The listing builds one solid part. Answer for the finished solid, in the listing's coordinates (mm). A direction names the side the tool comes from. Coordinates: 2 decimals unless noted, no trailing zeros. Write each loop counter-clockwise with the first axis right and the second up, starting at its lowest first coordinate (ties: lowest second). Pieces come first, ordered by that corner, then holes. Notation, with made-up numbers: M -7.75,9.25 L 33.25,9.25 A31 cw 33.25,43.25 Z; hole C 86,-35 d6. An arc over 180 degrees is marked long. Answer as a JSON object with one key per item and string values. Group by question number.
from build123d import *

# Parameters (mm, degrees)
F0_W      = 140
F0_H      = 70
F1_DEPTH  = 37
F2_W      = 138
F2_H      = 35
F3_DEPTH  = 70.001
F5_D      = 3.3
F6_W      = 2
F6_H      = 35
F7_DEPTH  = 35
F8_SIZE   = 34.99999
F10_DEPTH = 70.001
F11_W     = 60
F11_H     = 13
F12_DEPTH = 2.001
F13_W     = 33.65
F13_H     = 21.7
F13_W_2   = 26.7
F13_H_2   = 19.15
F13_W_3   = 30.8
F13_W_4   = 16.7
F13_W_5   = 22.15
F14_DEPTH = 2.001
F15_R     = 5
F17_D     = 4.4


# Not quite as in the source:
# - a fillet or chamfer is up to 0.001 mm smaller than in the source, because OpenCascade refuses the exact size
# - a feature names something its author has since deleted; it is built from what else it names


with BuildPart() as f1:
    # F0 (on Top) → F1 (new body)
    with BuildSketch(Plane.XY):
        with Locations((-10, 0)):
            Rectangle(F0_W, F0_H)
    extrude(amount=F1_DEPTH)

    # F2 (on face) → F3 (cut, through all)
    with BuildSketch(Plane.XZ.offset(35)):
        with Locations((-11, 19.5)):
            Rectangle(F2_W, F2_H)
    extrude(amount=-F3_DEPTH, mode=Mode.SUBTRACT)

    # F5 (through all)
    with Locations(Plane.XY.offset(2)):
        with Locations((-67, 25), (-59.5, 17.5), (-67, -25), (-59.5, -17.5), (-29.5, -17.5), (-22, -25), (-12, -20), (-12, 20), (-22, 25), (-29.5, 17.5), (28, 20), (38, 20), (38, -20), (28, -20)):
            Hole(F5_D / 2)

    # F6 (on face) → F7 (join)
    with BuildSketch(Plane(origin=(58, 0, 0), x_dir=(0, -1, 0), z_dir=(-1, 0, 0))):
        with Locations((-34, 19.5)):
            Rectangle(F6_W, F6_H)
        with Locations((34, 19.5)):
            Rectangle(F6_W, F6_H)
    extrude(amount=F7_DEPTH)

    # F8 (size 35 in the source; OpenCascade refuses exactly that, so slightly less here)
    f8_edges = [f1.edges().sort_by_distance(p)[0] for p in [
        (23, -34, 37),
        (23, 34, 37),
    ]]
    chamfer(f8_edges, length=F8_SIZE)

    # F9 (on face) → F10 (cut, through all)
    with BuildSketch(Plane.XZ.offset(35)):
        Polygon((58, 2), (58, 29.9289321881), (30.0710678119, 2), align=None)
    extrude(amount=-F10_DEPTH, mode=Mode.SUBTRACT)

    # F11 (on face) → F12 (cut, through all)
    with BuildSketch(Plane(origin=(58, 0, 0), x_dir=(0, -1, 0), z_dir=(-1, 0, 0))):
        with Locations((0, 8.5)):
            Rectangle(F11_W, F11_H)
    extrude(amount=-F12_DEPTH, mode=Mode.SUBTRACT)

    # F13 (on face) → F14 (cut, through all)
    with BuildSketch(Plane.XY.offset(2)):
        with Locations((38.175, 0)):
            Rectangle(F13_W, F13_H)
        with Locations((8, 0)):
            Rectangle(F13_W_2, F13_H)
        with Locations((8, 20.425)):
            Rectangle(F13_W_2, F13_H_2)
        with Locations((-20.75, 0)):
            Rectangle(F13_W_3, F13_H)
        with Locations((8, -20.425)):
            Rectangle(F13_W_2, F13_H_2)
        with Locations((-44.5, 0)):
            Rectangle(F13_W_4, F13_H)
        with Locations((-44.5, 20.425)):
            Rectangle(F13_W_4, F13_H_2)
        with Locations((-63.925, 0)):
            Rectangle(F13_W_5, F13_H)
        with Locations((-44.5, -20.425)):
            Rectangle(F13_W_4, F13_H_2)
    extrude(amount=-F14_DEPTH, mode=Mode.SUBTRACT)

    # F15 (call 1 of 28: OpenCascade refuses the feature's edges together)
    f15_edges = [f1.edges().sort_by_distance(p)[0] for p in [
        (55, 10.85, 1),
    ]]
    fillet(f15_edges, radius=F15_R)

    # F15#2 (call 2 of 28)
    f15_2_edges = [f1.edges().sort_by_distance(p)[0] for p in [
        (55, -10.85, 1),
    ]]
    fillet(f15_2_edges, radius=F15_R)

    # F15#3 (call 3 of 28)
    f15_3_edges = [f1.edges().sort_by_distance(p)[0] for p in [
        (21.35, -10.85, 1),
    ]]
    fillet(f15_3_edges, radius=F15_R)

    # F15#4 (call 4 of 28)
    f15_4_edges = [f1.edges().sort_by_distance(p)[0] for p in [
        (21.35, 10.85, 1),
    ]]
    fillet(f15_4_edges, radius=F15_R)

    # F15#5 (call 5 of 28)
    f15_5_edges = [f1.edges().sort_by_distance(p)[0] for p in [
        (21.35, -30, 1),
    ]]
    fillet(f15_5_edges, radius=F15_R)

    # F15#6 (call 6 of 28)
    f15_6_edges = [f1.edges().sort_by_distance(p)[0] for p in [
        (21.35, 30, 1),
    ]]
    fillet(f15_6_edges, radius=F15_R)

    # F15#7 (call 7 of 28)
    f15_7_edges = [f1.edges().sort_by_distance(p)[0] for p in [
        (-5.35, -30, 1),
    ]]
    fillet(f15_7_edges, radius=F15_R)

    # F15#8 (call 8 of 28)
    f15_8_edges = [f1.edges().sort_by_distance(p)[0] for p in [
        (-5.35, -10.85, 1),
    ]]
    fillet(f15_8_edges, radius=F15_R)

    # F15#9 (call 9 of 28)
    f15_9_edges = [f1.edges().sort_by_distance(p)[0] for p in [
        (-5.35, 10.85, 1),
    ]]
    fillet(f15_9_edges, radius=F15_R)

    # F15#10 (call 10 of 28)
    f15_10_edges = [f1.edges().sort_by_distance(p)[0] for p in [
        (-5.35, 30, 1),
    ]]
    fillet(f15_10_edges, radius=F15_R)

    # F15#11 (call 11 of 28)
    f15_11_edges = [f1.edges().sort_by_distance(p)[0] for p in [
        (-36.15, 10.85, 1),
    ]]
    fillet(f15_11_edges, radius=F15_R)

    # F15#12 (call 12 of 28)
    f15_12_edges = [f1.edges().sort_by_distance(p)[0] for p in [
        (-36.15, -30, 1),
    ]]
    fillet(f15_12_edges, radius=F15_R)

    # F15#13 (call 13 of 28)
    f15_13_edges = [f1.edges().sort_by_distance(p)[0] for p in [
        (-36.15, -10.85, 1),
    ]]
    fillet(f15_13_edges, radius=F15_R)

    # F15#14 (call 14 of 28)
    f15_14_edges = [f1.edges().sort_by_distance(p)[0] for p in [
        (-36.15, 30, 1),
    ]]
    fillet(f15_14_edges, radius=F15_R)

    # F15#15 (call 15 of 28)
    f15_15_edges = [f1.edges().sort_by_distance(p)[0] for p in [
        (-52.85, -30, 1),
    ]]
    fillet(f15_15_edges, radius=F15_R)

    # F15#16 (call 16 of 28)
    f15_16_edges = [f1.edges().sort_by_distance(p)[0] for p in [
        (-52.85, -10.85, 1),
    ]]
    fillet(f15_16_edges, radius=F15_R)

    # F15#17 (call 17 of 28)
    f15_17_edges = [f1.edges().sort_by_distance(p)[0] for p in [
        (-75, -10.85, 1),
    ]]
    fillet(f15_17_edges, radius=F15_R)

    # F15#18 (call 18 of 28)
    f15_18_edges = [f1.edges().sort_by_distance(p)[0] for p in [
        (-52.85, 10.85, 1),
    ]]
    fillet(f15_18_edges, radius=F15_R)

    # F15#19 (call 19 of 28)
    f15_19_edges = [f1.edges().sort_by_distance(p)[0] for p in [
        (-75, 10.85, 1),
    ]]
    fillet(f15_19_edges, radius=F15_R)

    # F15#20 (call 20 of 28)
    f15_20_edges = [f1.edges().sort_by_distance(p)[0] for p in [
        (-52.85, 30, 1),
    ]]
    fillet(f15_20_edges, radius=F15_R)

    # F15#21 (call 21 of 28)
    f15_21_edges = [f1.edges().sort_by_distance(p)[0] for p in [
        (30.071068, -34, 2),
    ]]
    fillet(f15_21_edges, radius=F15_R)

    # F15#22 (call 22 of 28)
    f15_22_edges = [f1.edges().sort_by_distance(p)[0] for p in [
        (30.071068, 34, 2),
    ]]
    fillet(f15_22_edges, radius=F15_R)

    # F15#23 (call 23 of 28)
    f15_23_edges = [f1.edges().sort_by_distance(p)[0] for p in [
        (58, 32.5, 2),
        (59, 30, 2),
    ]]
    fillet(f15_23_edges, radius=F15_R)

    # F15#24 (call 24 of 28)
    f15_24_edges = [f1.edges().sort_by_distance(p)[0] for p in [
        (58, 34, 29.928932),
    ]]
    fillet(f15_24_edges, radius=F15_R)

    # F15#25 (call 25 of 28)
    f15_25_edges = [f1.edges().sort_by_distance(p)[0] for p in [
        (58, -32.5, 2),
        (59, -30, 2),
    ]]
    fillet(f15_25_edges, radius=F15_R)

    # F15#26 (call 26 of 28)
    f15_26_edges = [f1.edges().sort_by_distance(p)[0] for p in [
        (58, -34, 29.928932),
    ]]
    fillet(f15_26_edges, radius=F15_R)

    # F15#27 (call 27 of 28)
    f15_27_edges = [f1.edges().sort_by_distance(p)[0] for p in [
        (59, -30, 15),
    ]]
    fillet(f15_27_edges, radius=F15_R)

    # F15#28 (call 28 of 28)
    f15_28_edges = [f1.edges().sort_by_distance(p)[0] for p in [
        (59, 30, 15),
    ]]
    fillet(f15_28_edges, radius=F15_R)

    # F17 (through all)
    with Locations(Plane.YZ.offset(60)):
        with Locations((-8, 32), (8, 32), (-8, 19), (8, 19)):
            Hole(F17_D / 2)


solid = f1.part
Item 1: A cutting plane is placed at D-D, the plane z = 32. Write down the section's boundary in (x, y), and give its area (3 significant figures).
Item 2: A cutting plane is placed at A-A, the plane x = -67. Write down the section's boundary in (y, z).
Item 3: A cutting plane is placed at C-C, the plane y = 8. Write down the section's boundary in (x, z).
Item 4: A cutting plane is placed at B-B, the plane x = 14. Write down the section's boundary in (y, z).
Item 5: Flat-ended cylindrical pins translate along their axes: pin 1 Ø5 at (y, z) = (8, 32) entering from -X; pin 2 Ø4 at (x, y) = (28, 20) entering from +Z. Find the tip coordinate at first contact, or state that the pin passes through.
Item 6: A tool of negligible diameter and unlimited length cuts with its end or side. For faces 3 (the face through (54.989, -33.986, 22.445)), 4 (the face through (58, -28, 3)), 5 (the face through (16, -35, 1)), 6 (the face through (53.57, 9.35, 0.99)), from which of +Z, -Z, +X, -X, +Y, -Y can it reach the whole face along a straight path? Write none if from no direction.
Item 7: For a pull along X with two mould halves and no side action, classify faces 1 (the face through (-20.784, -23.885, 0.986)), 2 (the face through (58.986, 8.477, 16.852)) as +X half, -X half, draft (parallel to the pull), parting line (faces both ways), or undercut.
Item 8: Consider L1, parallel to Y at x = 38, z = 1.5; L2, parallel to Z at x = -29, y = -29.5; L3, parallel to X at y = -21, z = 27. Determine where each line is inside the solid, lowest interval first. Write a range as from..to.
Answer:
{
 "1": {"outline": "M 53,-35 L 60,-35 L 60,-10.2 L 58,-10.2 L 58,-33 L 53,-33 Z; M 53,33 L 58,33 L 58,10.2 L 60,10.2 L 60,35 L 53,35 Z; M 58,-5.8 L 60,-5.8 L 60,5.8 L 58,5.8 Z", "area": "142 mm2"},
 "2": {"outline": "M -35,0 L -26.65,0 L -26.65,2 L -35,2 Z; M -23.35,0 L -10.85,0 L -10.85,2 L -23.35,2 Z; M 10.85,0 L 23.35,0 L 23.35,2 L 10.85,2 Z; M 26.65,0 L 35,0 L 35,2 L 26.65,2 Z"},
 "3": {"outline": "M -80,0 L -74.51,0 L -74.51,2 L -80,2 Z; M 54.51,0 L 60,0 L 60,2 L 54.51,2 Z; M 58,15 L 60,15 L 60,16.8 L 58,16.8 Z; M 58,21.2 L 60,21.2 L 60,29.8 L 58,29.8 Z; M 58,34.2 L 60,34.2 L 60,37 L 58,37 Z"},
 "4": {"outline": "M -35,0 L -30,0 L -30,2 L -35,2 Z; M 30,0 L 35,0 L 35,2 L 30,2 Z"},
 "5": {"pin 1": "x = 58", "pin 2": "z = 2"},
 "6": {"face 3": "+Y, -Y", "face 4": "+X, -X", "face 5": "+Z, -Z, +X, -X, -Y", "face 6": "+Z, -Z"},
 "7": {"face 1": "undercut", "face 2": "draft"},
 "8": {"L1": "-35..-21.65, -18.35..-10.85, 10.85..18.35, 21.65..35", "L2": "0..2", "L3": "58..60"}
}
